```python
from build123d import *

# Parameters (mm, degrees)
ESQUISSE1_W        = 240
ESQUISSE1_H        = 40
BOSS_EXTRU_1_DEPTH = 2
CONG_1_R           = 20


with BuildPart() as part:
    # Esquisse1 → Boss.-Extru.1 (new body)
    with BuildSketch(Plane.XY):
        Polygon((-610.5, 0), (610.5, 0), (610.5, 120), (45, 120), (45, 60), (-45, 60), (-45, 120), (-610.5, 120), (-668.615113653, 120), (-668.615113653, 60), (-968.615113653, 60), (-968.615113653, 0), align=None)
        with Locations((292.5, 40)):
            Rectangle(ESQUISSE1_W, ESQUISSE1_H, mode=Mode.SUBTRACT)
        with Locations((-292.5, 40)):
            Rectangle(ESQUISSE1_W, ESQUISSE1_H, mode=Mode.SUBTRACT)
    extrude(amount=BOSS_EXTRU_1_DEPTH)

    # Congé1
    cong_1_edges = [part.edges().sort_by_distance(p)[0] for p in [
        (-968.615113653, 60, 1),
        (-668.615113653, 60, 1),
        (-668.615113653, 120, 1),
    ]]
    fillet(cong_1_edges, radius=CONG_1_R)


solid = part.part
```
Here's how the part is built. I have some questions about the finished solid (model axes, mm). Round coordinates to 2 decimals unless told otherwise and drop trailing zeros. Write each loop counter-clockwise with the first axis right and the second up, starting at its lowest first coordinate (ties: lowest second). Pieces come first, ordered by that corner, then holes. Notation, with made-up numbers: M 34,-39.5 L 71,-39.5 A31 ccw 71,-10.5 Z; hole C 24.5,-0.75 d9. An arc over 180 degrees is marked long. Answer as CSV lines item,"result". Start each with the question number.
1. I need wall thicknesses on probe 1 along X at (y, z) = (38.5, 1.85); probe 2 along Y at (x, z) = (239, 1.2); probe 3 along X at (y, z) = (50.5, 0.3). Which ranges of each line are inside material? Lowest first, please.
2. Suppose I cut it at C-C on x = -23. Write out the boundary of the cut face in (y, z), then the cut area to 3 significant figures.
3. Suppose I cut it at A-A on x = -272. Write out the boundary of the cut face in (y, z).
4. Suppose I cut it at B-B on z = 1.1. Write out the boundary of the cut face in (x, y), then the cut area to 3 significant figures.
5. I'm going to push flat-ended pins straight in: pin 1 Ø0.6 at (x, z) = (-883, 0.5) entering from +Y; pin 2 Ø0.6 at (y, z) = (89.5, 1) entering from -X. Where does each tip first touch, or does it pass through?
Check result:
1,probe 1,"x = -968.62 to -412.5, -172.5 to 172.5, 412.5 to 610.5"
1,probe 2,"y = 0 to 20, 60 to 120"
1,probe 3,"x = -965.64 to -412.5, -172.5 to 172.5, 412.5 to 610.5"
2,outline,"M 0,0 L 60,0 L 60,2 L 0,2 Z"
2,area,"120 mm2"
3,outline,"M 0,0 L 20,0 L 20,2 L 0,2 Z; M 60,0 L 120,0 L 120,2 L 60,2 Z"
4,outline,"M -968.62,0 L 610.5,0 L 610.5,120 L 45,120 L 45,60 L -45,60 L -45,120 L -648.62,120 A20 ccw -668.62,100 L -668.62,80 A20 cw -688.62,60 L -948.62,60 A20 ccw -968.62,40 Z; hole M -412.5,20 L -172.5,20 L -172.5,60 L -412.5,60 Z; hole M 172.5,20 L 412.5,20 L 412.5,60 L 172.5,60 Z"
4,area,"147,000 mm2"
5,pin 1,"stops at y = 60"
5,pin 2,"stops at x = -668.62"
